from build123d import *

# Parameters (mm, degrees)
BOSS_EXTRUDE1_DEPTH      = 2
FILLET1_R                = 0.5
SKETCH2_R                = 9
BOSS_EXTRUDE2_DEPTH      = 1
SKETCH3_R                = 8.5
BOSS_EXTRUDE3_DEPTH      = 4
CUT_EXTRUDE1_DEPTH       = 16.375249198
BOSS_EXTRUDE4_DEPTH      = 1
BOSS_EXTRUDE4_DEPTH_BACK = 1
SKETCH5_R                = 8.5
SKETCH6_R                = 8.5
BOSS_EXTRUDE5_DEPTH      = 1
CHAMFER2_SIZE            = 1
SKETCH7_R                = 2.1
CUT_EXTRUDE2_DEPTH       = 2
CHAMFER3_SIZE            = 0.2


with BuildPart() as part:
    # Sketch1 → Boss-Extrude1 (new body)
    with BuildSketch(Plane(origin=(0, 31, 0), x_dir=(1, 0, 0), z_dir=(0, 1, 0))):
        Polygon((0, 10.392304845), (-9, 5.196152423), (-9, -5.196152423), (0, -10.392304845), (9, -5.196152423), (9, 5.196152423), align=None)
    extrude(amount=BOSS_EXTRUDE1_DEPTH)

    # Fillet1
    fillet1_edges = [part.edges().sort_by_distance(p)[0] for p in [
        (9, 32, -5.196152423),
        (9, 32, 5.196152423),
        (0, 32, 10.392304845),
        (-9, 32, 5.196152423),
        (-9, 32, -5.196152423),
        (0, 32, -10.392304845),
    ]]
    fillet(fillet1_edges, radius=FILLET1_R)

    # Sketch2 → Boss-Extrude2 (add)
    with BuildSketch(Plane(origin=(0, 33, 0), x_dir=(1, 0, 0), z_dir=(0, 1, 0))):
        with Locations(Location((0, 0, 0), (0, 0, 60))):
            Circle(SKETCH2_R)
    extrude(amount=BOSS_EXTRUDE2_DEPTH)

    # Sketch3 → Boss-Extrude3 (add)
    with BuildSketch(Plane(origin=(0, 34, 0), x_dir=(1, 0, 0), z_dir=(0, 1, 0))):
        with Locations(Location((0, 0, 0), (0, 0, 270))):
            Circle(SKETCH3_R)
    extrude(amount=BOSS_EXTRUDE3_DEPTH)

    # Sketch4 → Cut-Extrude1 (cut, through all)
    with BuildSketch(Plane(origin=(0, 38, 0), x_dir=(1, 0, 0), z_dir=(0, 1, 0))):
        Polygon((0, 2.886751346), (-2.5, 1.443375673), (-2.5, -1.443375673), (0, -2.886751346), (2.5, -1.443375673), (2.5, 1.443375673), align=None)
    extrude(amount=-CUT_EXTRUDE1_DEPTH, mode=Mode.SUBTRACT)

    # Sketch5 → Boss-Extrude4 (add, two sides: drawn at the far end of the back side and taken through both)
    with BuildSketch(Plane(origin=(0, 38, 0), x_dir=(1, 0, 0), z_dir=(0, 1, 0)).offset(-BOSS_EXTRUDE4_DEPTH_BACK)):
        with Locations(Location((0, 0, 0), (0, 0, 270))):
            Circle(SKETCH5_R)
    extrude(amount=BOSS_EXTRUDE4_DEPTH + BOSS_EXTRUDE4_DEPTH_BACK)

    # Sketch6 → Boss-Extrude5 (add)
    with BuildSketch(Plane(origin=(0, 39, 0), x_dir=(1, 0, 0), z_dir=(0, 1, 0))):
        with Locations(Location((0, 0, 0), (0, 0, 270))):
            Circle(SKETCH6_R)
    extrude(amount=BOSS_EXTRUDE5_DEPTH)

    # Chamfer2
    chamfer2_edges = [part.edges().sort_by_distance(p)[0] for p in [
        (0, 40, -8.5),
    ]]
    chamfer(chamfer2_edges, length=CHAMFER2_SIZE)

    # Sketch7 → Cut-Extrude2 (cut)
    with BuildSketch(Plane(origin=(0, 40, 0), x_dir=(1, 0, 0), z_dir=(0, 1, 0))):
        with Locations(Location((0, 0, 0), (0, 0, 270))):
            Circle(SKETCH7_R)
    extrude(amount=-CUT_EXTRUDE2_DEPTH, mode=Mode.SUBTRACT)

    # Chamfer3
    chamfer3_edges = [part.edges().sort_by_distance(p)[0] for p in [
        (0, 40, -2.1),
    ]]
    chamfer(chamfer3_edges, length=CHAMFER3_SIZE)


solid = part.part
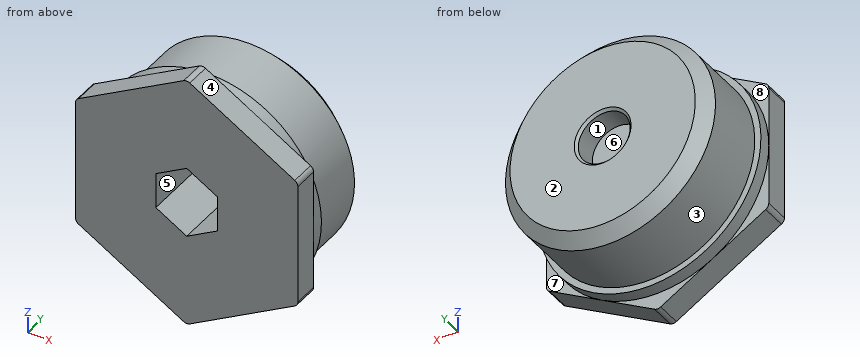
Can you work these out from the model? Positions are in its coordinate system, mm. Face numbers are marked on the shaded views. A direction names the side the tool comes from. Round coordinates to 2 decimals unless told otherwise and drop trailing zeros. Loops run counter-clockwise (first coordinate to the right, second up) from the corner with the lowest first, then second, coordinate; pieces in that order, holes last. Notation, with made-up numbers: (11, -5) - (27, -5) arc R25 cw to (27, 11) - close; hole circle Ø6 at (-12.75, -24). An arc over 180 degrees is marked (long way). Use CSV: the item, a comma, the result in double quotes. Start each with the question number.
1) If we section it at A-A on y = 32.75: Write out the boundary of the cut face in (x, z), plus the area to 3 significant figures.
2) For pin 1 Ø1 at (y, z) = (35.5, -2.5) entering from -X; pin 2 Ø4 at (x, z) = (0, 0) entering from +Y; pin 3 Ø3 at (x, y) = (-3.5, 33) entering from +Z; pin 4 Ø1.4 at (y, z) = (34.5, 0.5) entering from +X, each with a flat end and sliding along its axis, tell me the tip position at first contact or that it passes through.
3) Please list where these lines run through material, in increasing order: probe 1 along X at (y, z) = (38.85, 0); probe 2 along Y at (x, z) = (0.5, 0.25); probe 3 along X at (y, z) = (39.35, 0). Write a range as [from, to].
4) For the marked faces 5, 6, 7 and 8, which set-ups out of +Z, -Z, +X, -X, +Y, -Y let a thin tool reach every point of the face, with its end or its side?
5) We'd pull the mould along X, two halves only. Please class the marked faces 1, 2, 3 and 4: released by +X, released by -X, zero draft, split by the parting line, or undercut.
Geometry results:
1,outline,"(-9, -4.91) arc R0.5 ccw to (-8.75, -5.34) - (-0.25, -10.25) arc R0.5 ccw to (0.25, -10.25) - (8.75, -5.34) arc R0.5 ccw to (9, -4.91) - (9, 4.91) arc R0.5 ccw to (8.75, 5.34) - (0.25, 10.25) arc R0.5 ccw to (-0.25, 10.25) - (-8.75, 5.34) arc R0.5 ccw to (-9, 4.91) - close; hole (-2.5, -1.44) - (0, -2.89) - (2.5, -1.44) - (2.5, 1.44) - (0, 2.89) - (-2.5, 1.44) - close"
1,area,"259 mm2"
2,pin 1,"stops at x = -8.26"
2,pin 2,"stops at y = 38"
2,pin 3,"stops at z = 9.24"
2,pin 4,"stops at x = 9"
3,probe 1,"x = [-8.5, -2.1], [2.1, 8.5]"
3,probe 2,"y = [37, 38]"
3,probe 3,"x = [-8.15, -2.1], [2.1, 8.15]"
4,face 5,"-Y"
4,face 6,"+Y"
4,face 7,"-Z, +X, +Y"
4,face 8,"+Z, -X, +Y"
5,face 1,"undercut"
5,face 2,"zero draft"
5,face 3,"split by the parting line"
5,face 4,"released by +X"
